Here's how the part is built. I have some questions about the finished solid (model axes, mm). A direction names the side the tool comes from. Coordinates: 2 decimals unless noted, no trailing zeros. Write each loop counter-clockwise with the first axis right and the second up, starting at its lowest first coordinate (ties: lowest second). Pieces come first, ordered by that corner, then holes.
Item 1: Please list where these lines run through material, in increasing order: line 1 (X direction, y = 69, z = -2); line 2 (Y direction, x = 12.5, z = 0); line 3 (Y direction, x = 12, z = 5.5).
Item 2: If we mould it in two halves opening along Y, with no side actions, what happens to faces 6 (the face through (-15, 55, -12)), 7 (the face through (13, 0, -9)), 8 (the face through (1, 40, 2.85))? For each: pulls with the +Y half, pulls with the -Y half, needs draft (parallel to the pull), parting line crosses it, or undercut.
Item 3: I want a section at A-A (z = 4). Please give me the cut outline in (x, y).
Item 4: I'm going to push flat-ended pins straight in: P1, Ø1.9, axis at x = -5.5, y = 69, coming from the -Z side; P2, Ø12, axis at y = 18, z = -4.5, coming from the -X side; P3, Ø12, axis at y = 12.5, z = -3.5, coming from the -X side; P4, Ø3, axis at y = 24.5, z = -21.5, coming from the -X side. Where does each tip first touch, or does it pass through?
Item 5: For faces 1 (the face through (17.625, 25.304, 6.141)), 2 (the face through (0.67, 56.4, 6.14)), 3 (the face through (13.64, 7.05, -8.66)), 4 (the face through (10, 63, 9.525)), 5 (the face through (19, 42.5, 6)), which set-ups out of +Z, -Z, +X, -X, +Y, -Y let a thin tool reach every point of the face, with its end or its side?
Item 6: I want a section at C-C (x = 12.5). Please give me the cut outline in (y, z) (3 decimals), and give its area (3 significant figures).
Item 7: I want a section at D-D (x = -5.5). Please give me the cut outline in (y, z) (3 decimals).
Item 8: I want a section at B-B (z = -10). Please give me the cut outline in (x, y), and give its area (3 significant figures).
from build123d import *
from build123d.topology import SkipClean

# Parameters (mm, degrees)
SKETCH1_R           = 1.5
SKETCH1_W           = 15
SKETCH1_H           = 37.5
BOSS_EXTRUDE1_DEPTH = 2.85
FILLET1_R           = 5
FILLET2_R           = 2
BOSS_EXTRUDE2_START = 3.5
SKETCH5_R           = 1.5
BOSS_EXTRUDE2_DEPTH = 3.5
FILLET3_R           = 3.5
FILLET4_R           = 2
FILLET5_R           = 2
SKETCH6_R           = 1.5
CUT_EXTRUDE1_DEPTH  = 10
SKETCH8_R           = 1.5
BOSS_EXTRUDE3_DEPTH = 6.35
BOSS_EXTRUDE4_START = 3.175
SKETCH9_R           = 1.5
BOSS_EXTRUDE4_DEPTH = 3.175
SKETCH10_W          = 40
SKETCH10_H          = 15.399494937
SKETCH10_W_2        = 25
BOSS_EXTRUDE5_DEPTH = 6.675
CUT_EXTRUDE2_START  = -6.675
CUT_EXTRUDE2_DEPTH  = 6.675
BOSS_EXTRUDE6_START = -9.2
BOSS_EXTRUDE6_DEPTH = 9.2
FILLET6_R           = 7
BOSS_EXTRUDE7_DEPTH = 6.675
FILLET7_R           = 3
FILLET8_R           = 1.5
SKETCH14_R          = 1.5
CUT_EXTRUDE3_DEPTH  = 81.63507689
SKETCH15_R          = 1.55
CUT_EXTRUDE4_DEPTH  = 81.63507689
BOSS_EXTRUDE8_START = 20
SKETCH16_R          = 1.55
BOSS_EXTRUDE8_DEPTH = 20


# Read off the part's stored shape, not the designer's step: Cut-Extrude2
with BuildPart() as part:
    # Sketch1 → Boss-Extrude1 (new body)
    # profile 1 of 2: a face of its own
    with BuildSketch(Plane.XY):
        Polygon((0, 37.5), (0, 0), (25, 0), (25, 75), (0, 75), align=None)
        with Locations((12.5, 6)):
            Circle(SKETCH1_R, mode=Mode.SUBTRACT)
        with Locations((12.5, 37.5)):
            Circle(SKETCH1_R, mode=Mode.SUBTRACT)
        with Locations((12.5, 69)):
            Circle(SKETCH1_R, mode=Mode.SUBTRACT)
    # profile 2 of 2: a face of its own
    with BuildSketch(Plane.XY):
        with Locations((-7.5, 56.25)):
            Rectangle(SKETCH1_W, SKETCH1_H)
    extrude(amount=BOSS_EXTRUDE1_DEPTH)

    # Fillet1
    fillet1_edges = [part.edges().sort_by_distance(p)[0] for p in [
        (25, 75, 1.425),
        (25, 0, 1.425),
        (0, 0, 1.425),
        (0, 37.5, 1.425),
        (-15, 75, 1.425),
    ]]
    fillet(fillet1_edges, radius=FILLET1_R)

    # Fillet2
    fillet2_edges = [part.edges().sort_by_distance(p)[0] for p in [
        (-15, 37.5, 1.425),
    ]]
    fillet(fillet2_edges, radius=FILLET2_R)

    # Sketch5 → Boss-Extrude2 (add)
    # profile 1 of 2: a face of its own
    with BuildSketch(Plane.XY.offset(2.85).offset(BOSS_EXTRUDE2_START)):
        with BuildLine():
            Line((-15, 42.5), (10.428932188, 42.5))
            Line((10.428932188, 42.5), (21.464466094, 53.535533906))
            Line((21.464466094, 53.535533906), (25, 57.071067812))
            Line((25, 57.071067812), (25, 70))
            ThreePointArc((25, 70), (23.535533906, 73.535533906), (20, 75))
            Line((20, 75), (-10, 75))
            ThreePointArc((-10, 75), (-13.535533906, 73.535533906), (-15, 70))
            Line((-15, 70), (-15, 42.5))
        make_face()
        with Locations((12.5, 69)):
            Circle(SKETCH5_R, mode=Mode.SUBTRACT)
    # profile 2 of 2: a face of its own
    with BuildSketch(Plane.XY.offset(2.85).offset(BOSS_EXTRUDE2_START)):
        with BuildLine():
            Line((14.571067812, 32.5), (0, 17.928932188))
            Line((0, 17.928932188), (0, 5))
            ThreePointArc((0, 5), (1.464466094, 1.464466094), (5, 0))
            Line((5, 0), (20, 0))
            ThreePointArc((20, 0), (23.535533906, 1.464466094), (25, 5))
            Line((25, 5), (25, 32.5))
            Line((25, 32.5), (14.571067812, 32.5))
        make_face()
        with Locations((12.5, 6)):
            Circle(SKETCH5_R, mode=Mode.SUBTRACT)
    extrude(amount=-BOSS_EXTRUDE2_DEPTH)

    # Fillet3
    fillet3_edges = [part.edges().sort_by_distance(p)[0] for p in [
        (10.428932188, 42.5, 4.6),
        (14.571067812, 32.5, 4.6),
    ]]
    fillet(fillet3_edges, radius=FILLET3_R)

    # Fillet4
    fillet4_edges = [part.edges().sort_by_distance(p)[0] for p in [
        (-15, 42.5, 4.6),
    ]]
    fillet(fillet4_edges, radius=FILLET4_R)

    # Fillet5
    fillet5_edges = [part.edges().sort_by_distance(p)[0] for p in [
        (25, 57.071067812, 4.6),
        (25, 32.5, 4.6),
        (0, 17.928932188, 4.6),
    ]]
    fillet(fillet5_edges, radius=FILLET5_R)

    # Sketch6 → Cut-Extrude1 (cut)
    with BuildSketch(Plane.XY.offset(6.35)):
        with Locations((-5.5, 69)):
            Circle(SKETCH6_R)
    extrude(amount=-CUT_EXTRUDE1_DEPTH, mode=Mode.SUBTRACT)

    # Sketch8 → Boss-Extrude3 (add)
    with SkipClean():  # the faces are left unmerged after this step: merging them gives an invalid solid
        with BuildSketch(Plane(origin=(0, 0, 0), x_dir=(-1, 0, 0), z_dir=(0, 0, -1))):
            with BuildLine():
                ThreePointArc((0, 32.5), (1.464466094, 36.035533906), (5, 37.5))
                Line((5, 37.5), (13, 37.5))
                ThreePointArc((13, 37.5), (14.414213562, 38.085786438), (15, 39.5))
                Line((15, 39.5), (15, 70))
                ThreePointArc((15, 70), (13.535533906, 73.535533906), (10, 75))
                Line((10, 75), (-20, 75))
                ThreePointArc((-20, 75), (-23.535533906, 73.535533906), (-25, 70))
                Line((-25, 70), (-25, 5))
                ThreePointArc((-25, 5), (-23.535533906, 1.464466094), (-20, 0))
                Line((-20, 0), (-5, 0))
                ThreePointArc((-5, 0), (-1.464466094, 1.464466094), (0, 5))
                Line((0, 5), (0, 32.5))
            make_face()
            with Locations((-12.5, 6)):
                Circle(SKETCH8_R, mode=Mode.SUBTRACT)
            with Locations((-12.5, 69)):
                Circle(SKETCH8_R, mode=Mode.SUBTRACT)
            with Locations((-12.5, 37.5)):
                Circle(SKETCH8_R, mode=Mode.SUBTRACT)
            with Locations(Location((5.5, 69, 0), (0, 0, 180))):
                Circle(SKETCH8_R, mode=Mode.SUBTRACT)
        extrude(amount=BOSS_EXTRUDE3_DEPTH)
    add(part.part.scale(1), mode=Mode.REPLACE)  # the faces are merged on a copy

    # Sketch9 → Boss-Extrude4 (add)
    # profile 1 of 2: a face of its own
    with BuildSketch(Plane.XY.offset(6.35).offset(BOSS_EXTRUDE4_START)):
        with BuildLine():
            ThreePointArc((16.02081528, 32.5), (14.681423267, 32.233578364), (13.545941546, 31.474873734))
            Line((13.545941546, 31.474873734), (0.585786438, 18.514718626))
            ThreePointArc((0.585786438, 18.514718626), (0.152240935, 17.865871928), (0, 17.100505063))
            Line((0, 17.100505063), (0, 5))
            ThreePointArc((0, 5), (1.464466094, 1.464466094), (5, 0))
            Line((5, 0), (20, 0))
            ThreePointArc((20, 0), (23.535533906, 1.464466094), (25, 5))
            Line((25, 5), (25, 30.5))
            ThreePointArc((25, 30.5), (24.414213562, 31.914213562), (23, 32.5))
            Line((23, 32.5), (16.02081528, 32.5))
        make_face()
    # profile 2 of 2: a face of its own
    with BuildSketch(Plane.XY.offset(6.35).offset(BOSS_EXTRUDE4_START)):
        with BuildLine():
            ThreePointArc((8.97918472, 42.5), (10.318576733, 42.766421636), (11.454058454, 43.525126266))
            Line((11.454058454, 43.525126266), (24.414213562, 56.485281374))
            ThreePointArc((24.414213562, 56.485281374), (24.847759065, 57.134128072), (25, 57.899494937))
            Line((25, 57.899494937), (25, 70))
            ThreePointArc((25, 70), (23.535533906, 73.535533906), (20, 75))
            Line((20, 75), (-10, 75))
            ThreePointArc((-10, 75), (-13.535533906, 73.535533906), (-15, 70))
            Line((-15, 70), (-15, 44.5))
            ThreePointArc((-15, 44.5), (-14.414213562, 43.085786438), (-13, 42.5))
            Line((-13, 42.5), (8.97918472, 42.5))
        make_face()
        with Locations((-5.5, 69)):
            Circle(SKETCH9_R, mode=Mode.SUBTRACT)
        with Locations((12.5, 69)):
            Circle(SKETCH9_R, mode=Mode.SUBTRACT)
    extrude(amount=-BOSS_EXTRUDE4_DEPTH)

    # Sketch10 → Boss-Extrude5 (add)
    with SkipClean():  # the faces are left unmerged after this step: merging them gives an invalid solid
        with BuildSketch(Plane.XY.offset(9.525)):
            with Locations((5, 50.199747469)):
                Rectangle(SKETCH10_W, SKETCH10_H)
            with Locations((12.5, 24.800252531)):
                Rectangle(SKETCH10_W_2, SKETCH10_H)
        extrude(amount=-BOSS_EXTRUDE5_DEPTH)

    # Cut-Extrude2 outline → Cut-Extrude2 (cut)
    with SkipClean():  # the faces are left unmerged after this step: merging them gives an invalid solid
        with BuildSketch(Plane.XY.offset(9.525).offset(CUT_EXTRUDE2_START)):
            Polygon((25, 32.5), (10.428932188, 32.5), (25, 17.928932188), align=None)
            with BuildLine():
                Line((-15, 42.5), (14.571067812, 42.5))
                Line((14.571067812, 42.5), (-14.682437359, 71.75350517))
                ThreePointArc((-14.682437359, 71.75350517), (-14.919968841, 70.891014367), (-15, 70))
                Line((-15, 70), (-15, 42.5))
            make_face()
        extrude(amount=CUT_EXTRUDE2_DEPTH, mode=Mode.SUBTRACT)

    # Sketch12 → Boss-Extrude6 (add)
    with BuildSketch(Plane(origin=(0, 0, -6.35), x_dir=(-1, 0, 0), z_dir=(0, 0, -1)).offset(BOSS_EXTRUDE6_START)):
        with BuildLine():
            Line((0, 0), (14.867488321, 38.784117768))
            ThreePointArc((14.867488321, 38.784117768), (14.133189202, 37.852006604), (13, 37.5))
            Line((13, 37.5), (5, 37.5))
            ThreePointArc((5, 37.5), (1.464466094, 36.035533906), (0, 32.5))
            Line((0, 32.5), (0, 5))
            ThreePointArc((0, 5), (-1.464466094, 1.464466094), (-5, 0))
            Line((-5, 0), (0, 0))
        make_face()
    extrude(amount=BOSS_EXTRUDE6_DEPTH)

    # Fillet6
    fillet6_edges = [part.edges().sort_by_distance(p)[0] for p in [
        (0, 0, -1.75),
    ]]
    fillet(fillet6_edges, radius=FILLET6_R)

    # Sketch13 → Boss-Extrude7 (add)
    with SkipClean():  # the faces are left unmerged after this step: merging them gives an invalid solid
        with BuildSketch(Plane.XY.offset(9.525)):
            with BuildLine():
                Line((0, 32.5), (0, 5))
                ThreePointArc((0, 5), (1.464466094, 1.464466094), (5, 0))
                Line((5, 0), (4.813322939, 0))
                ThreePointArc((4.813322939, 0), (0.847160732, 1.232023115), (-1.722886185, 4.494412187))
                Line((-1.722886185, 4.494412187), (-12.458537109, 32.5))
                Line((-12.458537109, 32.5), (0, 32.5))
            make_face()
        extrude(amount=-BOSS_EXTRUDE7_DEPTH)

    # Fillet7
    fillet7_edges = [part.edges().sort_by_distance(p)[0] for p in [
        (25, 42.5, 6.1875),
        (14.571067812, 42.5, 6.1875),
        (-14.682437359, 71.75350517, 4.6),
        (10.428932188, 32.5, 6.1875),
        (25, 17.928932188, 6.1875),
    ]]
    fillet(fillet7_edges, radius=FILLET7_R)

    # Fillet8
    # the kernel refuses this fillet: 1.5 mm, written as the material it takes off along each edge
    with BuildSketch(Plane(origin=(-12.458537109, 32.5, 14.978612885), x_dir=(0.35794111613384066, -0.9337441605605148, 0), z_dir=(0, 0, -1))) as fillet8_piece_1:
        with BuildLine():
            CenterArc((FILLET8_R * 1.45429676938, -FILLET8_R), FILLET8_R, 90, 110.97380664)
            Line((FILLET8_R * 0.520552608823, -FILLET8_R * 1.35794111613), (0, 0))
            Line((0, 0), (FILLET8_R * 1.45429676938, 0))
        make_face()
    extrude(amount=12.128612885, mode=Mode.SUBTRACT)

    # Sketch14 → Cut-Extrude3 (cut, through all)
    with SkipClean():  # the faces are left unmerged after this step: merging them gives an invalid solid
        with BuildSketch(Plane(origin=(0, 0, -6.35), x_dir=(-1, 0, 0), z_dir=(0, 0, -1))):
            with Locations((-12.5, 6)):
                Circle(SKETCH14_R)
        extrude(amount=-CUT_EXTRUDE3_DEPTH, mode=Mode.SUBTRACT)
    add(part.part.scale(1), mode=Mode.REPLACE)  # the faces are merged on a copy

    # Sketch15 → Cut-Extrude4 (cut, through all)
    with BuildSketch(Plane(origin=(0, 0, -6.35), x_dir=(-1, 0, 0), z_dir=(0, 0, -1))):
        with Locations((-12.5, 69)):
            Circle(SKETCH15_R)
        with Locations((5.5, 69)):
            Circle(SKETCH15_R)
        with Locations((-12.5, 37.5)):
            Circle(SKETCH15_R)
        with Locations((-12.5, 6)):
            Circle(SKETCH15_R)
    extrude(amount=-CUT_EXTRUDE4_DEPTH, mode=Mode.SUBTRACT)

    # Sketch16 → Boss-Extrude8 (add)
    with BuildSketch(Plane(origin=(0, 0, -6.35), x_dir=(-1, 0, 0), z_dir=(0, 0, -1)).offset(BOSS_EXTRUDE8_START)):
        with BuildLine():
            Line((-20, 0), (-4.813322939, 0))
            ThreePointArc((-4.813322939, 0), (-0.847160732, 1.232023115), (1.722886185, 4.494412187))
            Line((1.722886185, 4.494412187), (14.867488321, 38.784117768))
            ThreePointArc((14.867488321, 38.784117768), (14.966593075, 39.135978464), (15, 39.5))
            Line((15, 39.5), (15, 70))
            ThreePointArc((15, 70), (13.535533906, 73.535533906), (10, 75))
            Line((10, 75), (-20, 75))
            ThreePointArc((-20, 75), (-23.535533906, 73.535533906), (-25, 70))
            Line((-25, 70), (-25, 5))
            ThreePointArc((-25, 5), (-23.535533906, 1.464466094), (-20, 0))
        make_face()
        with Locations((-12.5, 6)):
            Circle(SKETCH16_R, mode=Mode.SUBTRACT)
        with Locations((-12.5, 37.5)):
            Circle(SKETCH16_R, mode=Mode.SUBTRACT)
        with Locations((5.5, 69)):
            Circle(SKETCH16_R, mode=Mode.SUBTRACT)
        with Locations((-12.5, 69)):
            Circle(SKETCH16_R, mode=Mode.SUBTRACT)
    extrude(amount=-BOSS_EXTRUDE8_DEPTH)


solid = part.part
Answer:
1. line 1: x = -15 to -7.05, -3.95 to 10.95, 14.05 to 25
1. line 2: y = 0 to 4.45, 7.55 to 35.95, 39.05 to 67.45, 70.55 to 75
1. line 3: y = 0 to 4.53, 7.47 to 30.93, 45.07 to 67.53, 70.47 to 75
2. face 6: needs draft
2. face 7: pulls with the -Y half
2. face 8: undercut
3. outline: (-12.72, 69.79) - (13.69, 43.38) arc R3 ccw to (15.81, 42.5) - (22, 42.5) arc R3 ccw to (25, 45.5) - (25, 70) arc R5 ccw to (20, 75) - (-10, 75) arc R5 ccw to (-11.49, 74.77) arc R3 ccw to start; (-11.68, 30.46) - (-1.72, 4.49) arc R7 ccw to (4.81, 0) - (20, 0) arc R5 ccw to (25, 5) - (25, 16.69) arc R3 ccw to (24.12, 18.81) - (11.31, 31.62) arc R3 ccw to (9.19, 32.5) - (-10.28, 32.5) arc R1.5 ccw to start; hole circle Ø3.1 at (-5.5, 69); hole circle Ø3.1 at (12.5, 6); hole circle Ø3.1 at (12.5, 69)
4. P1: passes through
4. P2: stops at x = -9.2
4. P3: stops at x = -7.09
4. P4: stops at x = -9.97
5. face 1: +Z, +X
5. face 2: +Z, -X
5. face 3: +Z, -Z
5. face 4: +Z, +X, -X, +Y, -Y
5. face 5: +Z, +X, -X
6. outline: (0, -26.35) - (4.45, -26.35) - (4.45, 9.525) - (0, 9.525) - close; (7.55, -26.35) - (35.95, -26.35) - (35.95, 2.85) - (30.429, 2.85) - (30.429, 9.525) - (7.55, 9.525) - close; (39.05, -26.35) - (67.45, -26.35) - (67.45, 9.525) - (44.571, 9.525) - (44.571, 2.85) - (39.05, 2.85) - close; (70.55, -26.35) - (75, -26.35) - (75, 9.525) - (70.55, 9.525) - close
6. area: 2,280 mm2
7. outline: (14.348, -26.35) - (67.45, -26.35) - (67.45, 9.525) - (62.571, 9.525) - (62.571, 2.85) - (32.5, 2.85) - (32.5, 9.525) - (14.348, 9.525) - close; (70.55, -26.35) - (75, -26.35) - (75, 9.525) - (70.55, 9.525) - close
8. outline: (-15, 39.5) arc R2 ccw to (-14.87, 38.78) - (-1.72, 4.49) arc R7 ccw to (4.81, 0) - (20, 0) arc R5 ccw to (25, 5) - (25, 70) arc R5 ccw to (20, 75) - (-10, 75) arc R5 ccw to (-15, 70) - close; hole circle Ø3.1 at (-5.5, 69); hole circle Ø3.1 at (12.5, 6); hole circle Ø3.1 at (12.5, 37.5); hole circle Ø3.1 at (12.5, 69)
8. area: 2,660 mm2
